For this review, take the finished solid that the model builds, in its own axes (mm). Round coordinates to 2 decimals unless told otherwise and drop trailing zeros. Write each loop counter-clockwise with the first axis right and the second up, starting at its lowest first coordinate (ties: lowest second). Pieces come first, ordered by that corner, then holes. Notation, with made-up numbers: M 3.25,45.5 L 14.25,45.5 A25 cw 14.25,62.5 Z; hole C -39,36.25 d3. An arc over 180 degrees is marked long. Use one line per item in the form item = value. Start each with the question number.
Item 1: Add section A-A (x = 0). State the section outline as (y, z) points, and give its area (3 significant figures).
Item 2: Draft analysis for pull direction X (two halves, no side actions). For faces 1 (the flat face through (0, 0, 0)), 2 (the cylindrical face through (0, -18, 4)), 3 (the cylindrical face through (-0.444, 12.999, 4.056)), 4 (the cylindrical face through (-0.444, -12.999, 4.056)), state which applies: released by +X, released by -X, zero draft, split by the parting line, or undercut.
Item 3: For P1, Ø2, axis at x = 2, z = 6, coming from the +Y side, flat-tipped, find the tip position at first contact; note if it passes through.
Item 4: For line 1 (Y direction, x = 0, z = 2); line 2 (Y direction, x = -1.4, z = 1.75); line 3 (X direction, y = 16.5, z = 0.75), list the stretches that pass through material, from the lowest coordinate up. Write a range as [from, to].
Item 5: Add section C-C (x = -2.5). State the section outline as (y, z) points.
Item 6: Add section B-B (z = 6.25). State the section outline as (x, y) points, and give its area (3 significant figures).
from build123d import *

# Parameters (mm, degrees)
BOSS_EXTRUDE1_DEPTH     = 8
F_4_0_MM_DOWEL_HOLES1_D = 4.1


with BuildPart() as part:
    # Sketch1 → Boss-Extrude1 (new body)
    with BuildSketch(Plane.XY):
        with BuildLine():
            Line((-3, 15), (-3, -15))
            ThreePointArc((-3, -15), (0, -18), (3, -15))
            Line((3, -15), (3, 15))
            ThreePointArc((3, 15), (0, 18), (-3, 15))
        make_face()
    extrude(amount=BOSS_EXTRUDE1_DEPTH)

    # Ø4.0 mm Dowel Holes1 (through all)
    with Locations(Plane(origin=(0, 0, 0), x_dir=(-1, 0, 0), z_dir=(0, 0, -1))):
        with Locations((0, 15)):
            f_4_0_mm_dowel_holes1 = Hole(F_4_0_MM_DOWEL_HOLES1_D / 2)

    # Mirror1: Ø4.0 mm Dowel Holes1 across plane
    add(f_4_0_mm_dowel_holes1.mirror(Plane.ZX), mode=Mode.SUBTRACT)


solid = part.part
Calculated:
q1.outline = M -18,0 L -17.05,0 L -17.05,8 L -18,8 Z; M -12.95,0 L 12.95,0 L 12.95,8 L -12.95,8 Z; M 17.05,0 L 18,0 L 18,8 L 17.05,8 Z
q1.area = 222 mm^2
q2.face_1 = zero draft
q2.face_2 = split by the parting line
q2.face_3 = undercut
q2.face_4 = undercut
q3.P1 = 17.83
q4.line_1 = [-18, -17.05], [-12.95, 12.95], [17.05, 18]
q4.line_2 = [-17.65, -16.5], [-13.5, 13.5], [16.5, 17.65]
q4.line_3 = [-2.6, -1.4], [1.4, 2.6]
q5.outline = M -16.66,0 L 16.66,0 L 16.66,8 L -16.66,8 Z
q6.outline = M -3,-15 A3 ccw 3,-15 L 3,15 A3 ccw -3,15 Z; hole C 0,-15 d4.1; hole C 0,15 d4.1
q6.area = 182 mm^2
